The model under review builds one solid part; all positions refer to its coordinate system, in mm. A direction names the side the tool comes from. Coordinates: 2 decimals unless noted, no trailing zeros. Write each loop counter-clockwise with the first axis right and the second up, starting at its lowest first coordinate (ties: lowest second). Pieces come first, ordered by that corner, then holes. Notation, with made-up numbers: (2, 66) - (37, 66) arc R20 cw to (37, 99) - close; hole circle Ø3 at (-40, -39.5). An arc over 180 degrees is marked (long way). Put each result on its own line as item: value. Start each with the question number.
Item 1: Consider section B-B on y = 458. Give the boundary of the cut face in (x, z) (3 decimals).
Item 2: To check wall thickness, follow L1, parallel to Y at x = 0, z = 6.65; L2, parallel to Z at x = -3, y = 322.5 (3 decimals). State the ranges of each line that lie inside material, in increasing order. Write a range as [from, to].
Item 3: Machinability: for faces 5 (the face through (0, 278, -6.055)), 6 (the face through (0, 271, -9.23)), which of the approach directions +Z, -Z, +X, -X, +Y, -Y give a long, thin tool a straight path to every point of the face, cutting with its end or side? Answer none if there is none.
Item 4: Consider section A-A on z = 0. Give the boundary of the cut face in (x, y) (3 decimals), then the cut area to 3 significant figures.
Item 5: Consider section C-C on x = 0. State how many separate pieces and enclosed holes the cut face has, then the cut area to 3 significant figures.
Item 6: For pin 1 (4 mm diameter, centred on x = 3.5, z = 5.5, fed in from +Y); pin 2 (9 mm diameter, centred on x = 0, y = 534.575, fed in from +Z); pin 3 (7 mm diameter, centred on x = 0, y = 518.675, fed in from +Z); pin 4 (4.5 mm diameter, centred on x = 0, y = 502.775, fed in from +Z), all flat-tipped, find the tip position at first contact; note any pin that passes through.
Item 7: Mouldability with a two-part tool opening along Z and no side actions: class faces 1 (the face through (-9.23, 271, 0)), 2 (the face through (-0.13, 531.68, 7.43)), 3 (the face through (7.113, 9.245, -0.127)), 4 (the face through (6.055, 278, 0)) as pulls with the +Z half, pulls with the -Z half, needs draft (parallel to the pull), parting line crosses it, or undercut.
```python
from build123d import *

# Parameters (mm, degrees)
SKETCH1_W           = 18.46
SKETCH1_H           = 18.46
SKETCH1_W_2         = 12.11
SKETCH1_H_2         = 12.11
BOSS_EXTRUDE1_DEPTH = 550.5
SKETCH2_W           = 12.11
SKETCH2_H           = 12.11
BOSS_EXTRUDE2_DEPTH = 12.7
LPATTERN1_COUNT     = 3
LPATTERN1_PITCH     = 15.9


with BuildPart() as part:
    # Sketch1 → Boss-Extrude1 (new body)
    with BuildSketch(Plane(origin=(0, 0, 0), x_dir=(1, 0, 0), z_dir=(0, 1, 0))):
        Rectangle(SKETCH1_W, SKETCH1_H)
        Rectangle(SKETCH1_W_2, SKETCH1_H_2, mode=Mode.SUBTRACT)
    extrude(amount=BOSS_EXTRUDE1_DEPTH)

    # Sketch2 → Boss-Extrude2 (add)
    with BuildSketch(Plane.XZ):
        Rectangle(SKETCH2_W, SKETCH2_H)
    extrude(amount=-BOSS_EXTRUDE2_DEPTH)

    # Sketch4 → Cut-Revolve1 (revolve, cut)
    with BuildSketch(Plane.XY):
        Polygon((-9.23, 6.365), (9.23, 6.365), (9.23, 1.365), (7.005, 3.59), (-9.23, 3.59), align=None)
    revolve(axis=Axis((-9.23, 6.365, 0), (1, 0, 0)), mode=Mode.SUBTRACT)

    # Sketch5 → Cut-Revolve2 (revolve, cut)
    with BuildSketch(Plane(origin=(0, 0, 0), x_dir=(0, 0, -1), z_dir=(1, 0, 0))):
        Polygon((-7.305, 537.35), (-9.23, 539.275), (-9.23, 534.575), (9.23, 534.575), (9.23, 537.35), align=None)
    cut_revolve2 = revolve(axis=Axis((0, 534.575, 9.23), (0, 0, 1)), mode=Mode.SUBTRACT)

    # LPattern1: Cut-Revolve2 ×3
    with Locations(*[(0, -i * LPATTERN1_PITCH, 0) for i in range(1, LPATTERN1_COUNT)]):
        add(cut_revolve2, mode=Mode.SUBTRACT)


solid = part.part
```
Report:
1. outline: (-9.23, -9.23) - (9.23, -9.23) - (9.23, 9.23) - (-9.23, 9.23) - close; hole (-6.055, -6.055) - (6.055, -6.055) - (6.055, 6.055) - (-6.055, 6.055) - close
2. L1: [0, 500], [505.55, 515.9], [521.45, 531.8], [537.35, 550.5]
2. L2: [-9.23, -6.055], [6.055, 9.23]
3. face 5: +Y
3. face 6: -Z, +X, -X, +Y, -Y
4. outline: (-9.23, 0) - (9.23, 0) - (9.23, 1.365) - (7.005, 3.59) - (-9.23, 3.59) - close; (-9.23, 9.14) - (7.005, 9.14) - (9.23, 11.365) - (9.23, 550.5) - (6.055, 550.5) - (6.055, 12.7) - (-6.055, 12.7) - (-6.055, 550.5) - (-9.23, 550.5) - close
4. area: 3,540 mm²
5. separate pieces: 7
5. enclosed holes: 1
5. area: 3,510 mm²
6. pin 1: y = 550.5
6. pin 2: z = 9.03
6. pin 3: z = 8.03
6. pin 4: through
7. face 1: needs draft
7. face 2: pulls with the +Z half
7. face 3: undercut
7. face 4: undercut
